The figure shows three views and two pictorial views of one solid part (mm, origin at its lowest corner). Answer the questions. A direction names the side the tool comes from. Round coordinates to 2 decimals unless told otherwise and drop trailing zeros. Order: outer loops, then holes, each group sorted by start corner. A loop starts at its lowest first (then second) coordinate and runs counter-clockwise, first axis right, second up. Notation, with made-up numbers: (80.25, -15.75) - (103.25, -15.75) arc R22 ccw to (103.25, 2.25) - close; hole circle Ø9 at (-36, 14.25). An arc over 180 degrees is marked (long way). One line per item, written item: value. Start each with the question number.
1. Section D-D, the plane y = 33 is taken. Give the vertices of the cut face in (x, z), then the cut area to 3 significant figures.
2. Straight lines are drawn through the part: line 1 (X direction, y = 5, z = 4.75); line 2 (Y direction, x = 16.5, z = 5.25). For each, find the intervals that lie inside material, in ascending order.
3. A tool of negligible diameter and unlimited length cuts with its end or side. For the marked faces 5, 6 and 7, from which of +Z, -Z, +X, -X, +Y, -Y can it reach the whole face along a straight path? Write none if from no direction.
4. For a pull along X with two mould halves and no side action, classify the marked faces 1, 2, 3 and 4 as released by +X, released by -X, zero draft, split by the parting line, or undercut.
5. A flat-ended cylindrical pin translates along its axis: P1, Ø3.5, axis at x = 45, y = 5, coming from the +Z side. Find the tip coordinate at first contact, or state that the pin passes through.
6. Section C-C, the plane z = 3.25 is taken. Give the vertices of the cut face in (x, y).
7. Section A-A, the plane y = 45 is taken. Give the vertices of the cut face in (x, z).
8. Section B-B, the plane x = 45 is taken. Give the vertices of the cut face in (y, z), then the cut area to 3 significant figures.
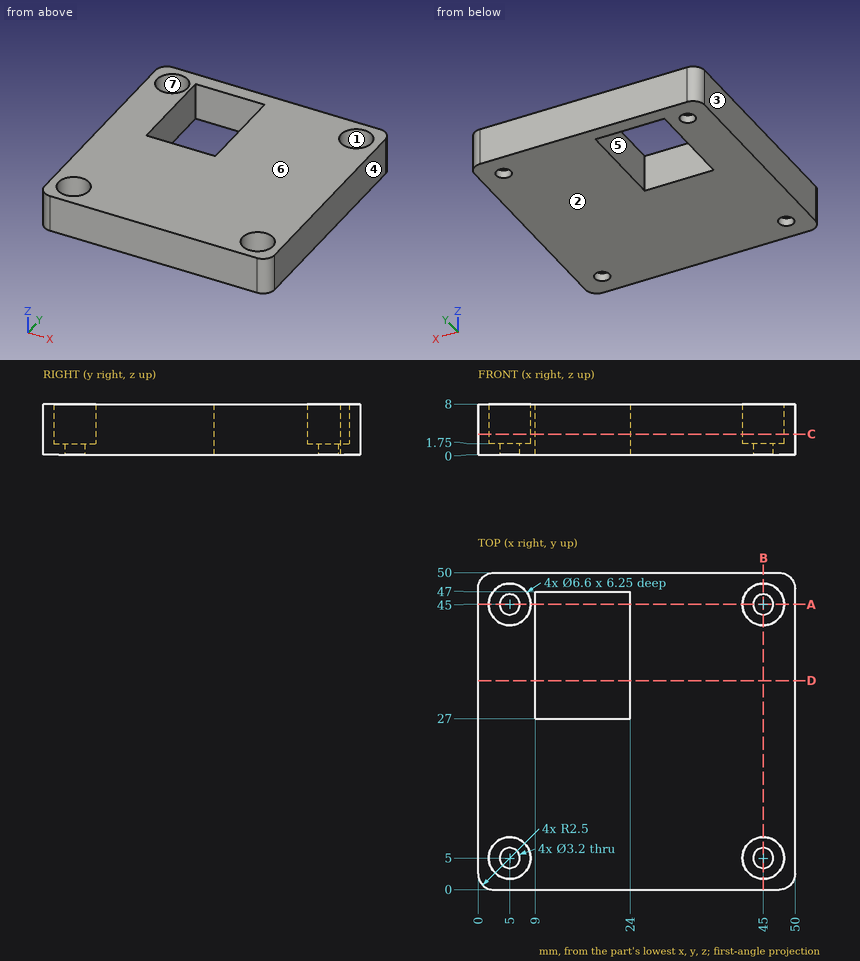
Answer list:
1. outline: (0, 0) - (9, 0) - (9, 8) - (0, 8) - close; (24, 0) - (50, 0) - (50, 8) - (24, 8) - close
1. area: 280 mm²
2. line 1: x = 0 to 1.7, 8.3 to 41.7, 48.3 to 50
2. line 2: y = 0 to 27, 47 to 50
3. face 5: +Z, -Z
3. face 6: +Z, +X, -X, +Y, -Y
3. face 7: +Z
4. face 1: undercut
4. face 2: zero draft
4. face 3: released by -X
4. face 4: released by +X
5. P1: stops at z = 1.75
6. outline: (0, 2.5) arc R2.5 ccw to (2.5, 0) - (47.5, 0) arc R2.5 ccw to (50, 2.5) - (50, 47.5) arc R2.5 ccw to (47.5, 50) - (2.5, 50) arc R2.5 ccw to (0, 47.5) - close; hole circle Ø6.6 at (5, 5); hole circle Ø6.6 at (5, 45); hole (9, 27) - (24, 27) - (24, 47) - (9, 47) - close; hole circle Ø6.6 at (45, 5); hole circle Ø6.6 at (45, 45)
7. outline: (0, 0) - (3.4, 0) - (3.4, 1.75) - (1.7, 1.75) - (1.7, 8) - (0, 8) - close; (6.6, 0) - (9, 0) - (9, 8) - (8.3, 8) - (8.3, 1.75) - (6.6, 1.75) - close; (24, 0) - (43.4, 0) - (43.4, 1.75) - (41.7, 1.75) - (41.7, 8) - (24, 8) - close; (46.6, 0) - (50, 0) - (50, 8) - (48.3, 8) - (48.3, 1.75) - (46.6, 1.75) - close
8. outline: (0, 0) - (3.4, 0) - (3.4, 1.75) - (1.7, 1.75) - (1.7, 8) - (0, 8) - close; (6.6, 0) - (43.4, 0) - (43.4, 1.75) - (41.7, 1.75) - (41.7, 8) - (8.3, 8) - (8.3, 1.75) - (6.6, 1.75) - close; (46.6, 0) - (50, 0) - (50, 8) - (48.3, 8) - (48.3, 1.75) - (46.6, 1.75) - close
8. area: 306 mm²
